from build123d import *

# Parameters (mm, degrees)
SKETCH_1_R          = 4
EXTRUDE_1_DEPTH     = 5
SKETCH_2_W          = 20.529114817
SKETCH_2_H          = 31.412366712
CUT_EXTRUDE_1_DEPTH = 5
EXTRUDE_2_DEPTH     = 20
SKETCH_4_W          = 7.585483435
SKETCH_4_H          = 20
EXTRUDE_3_DEPTH     = 10
SKETCH_5_W          = 7.585483435
SKETCH_5_H          = 20
SKETCH_5_W_2        = 3.706183356
EXTRUDE_4_DEPTH     = 5
SKETCH_6_W          = 3.75
SKETCH_6_H          = 12
CUT_EXTRUDE_2_DEPTH = 3
CUT_EXTRUDE_3_REACH = 54
SKETCH_7_R          = 1.275
FILLET_1_R          = 3
FILLET_2_R          = 1


with BuildPart() as part:
    # 草图1 → 凸台-拉伸1 (new body)
    with BuildSketch(Plane(origin=(0, 0, 0), x_dir=(1, 0, 0), z_dir=(0, 1, 0))):
        with BuildLine():
            Line((30, 40), (-30, 40))
            ThreePointArc((-30, 40), (-37.071067812, 37.071067812), (-40, 30))
            Line((-40, 30), (-40, -30))
            ThreePointArc((-40, -30), (-37.071067812, -37.071067812), (-30, -40))
            Line((-30, -40), (30, -40))
            ThreePointArc((30, -40), (37.071067812, -37.071067812), (40, -30))
            Line((40, -30), (40, 30))
            ThreePointArc((40, 30), (37.071067812, 37.071067812), (30, 40))
        make_face()
        with Locations((-30, 30)):
            Circle(SKETCH_1_R, mode=Mode.SUBTRACT)
        with Locations((-30, -30)):
            Circle(SKETCH_1_R, mode=Mode.SUBTRACT)
        with Locations((30, -30)):
            Circle(SKETCH_1_R, mode=Mode.SUBTRACT)
        with Locations((30, 30)):
            Circle(SKETCH_1_R, mode=Mode.SUBTRACT)
    extrude(amount=EXTRUDE_1_DEPTH)

    # 草图2 → 切除-拉伸1 (cut)
    with BuildSketch(Plane(origin=(0, 5, 0), x_dir=(1, 0, 0), z_dir=(0, 1, 0))):
        with Locations((-10.264557408, 0)):
            Rectangle(SKETCH_2_W, SKETCH_2_H)
    extrude(amount=-CUT_EXTRUDE_1_DEPTH, mode=Mode.SUBTRACT)

    # 草图3 → 凸台-拉伸2 (add)
    with BuildSketch(Plane(origin=(0, 5, 0), x_dir=(1, 0, 0), z_dir=(0, 1, 0))):
        with BuildLine():
            Line((0, -15.706183356), (-20.529114817, -15.706183356))
            Line((-20.529114817, -15.706183356), (-20.529114817, 15.706183356))
            Line((-20.529114817, 15.706183356), (0, 15.706183356))
            Line((0, 15.706183356), (0, 23.291666791))
            Line((0, 23.291666791), (-22.012764878, 23.291666791))
            ThreePointArc((-22.012764878, 23.291666791), (-25.548298784, 21.827200697), (-27.012764878, 18.291666791))
            Line((-27.012764878, 18.291666791), (-27.012764878, -18.291666791))
            ThreePointArc((-27.012764878, -18.291666791), (-25.548298784, -21.827200697), (-22.012764878, -23.291666791))
            Line((-22.012764878, -23.291666791), (0, -23.291666791))
            Line((0, -23.291666791), (0, -15.706183356))
        make_face()
    extrude(amount=EXTRUDE_2_DEPTH)

    # 草图4 → 凸台-拉伸3 (add)
    with BuildSketch(Plane(origin=(0, 0, 0), x_dir=(0, 0, -1), z_dir=(1, 0, 0))):
        with Locations((19.498925074, 15)):
            Rectangle(SKETCH_4_W, SKETCH_4_H)
        with Locations((-19.498925074, 15)):
            Rectangle(SKETCH_4_W, SKETCH_4_H)
    extrude(amount=EXTRUDE_3_DEPTH)

    # 草图5 → 凸台-拉伸4 (add, symmetric)
    with BuildSketch(Plane(origin=(10, 0, 0), x_dir=(0, 0, -1), z_dir=(1, 0, 0))):
        with Locations((-19.498925074, 15)):
            Rectangle(SKETCH_5_W, SKETCH_5_H)
        with Locations((-13.853091678, 15)):
            Rectangle(SKETCH_5_W_2, SKETCH_5_H)
        with Locations((13.853091678, 15)):
            Rectangle(SKETCH_5_W_2, SKETCH_5_H)
        with Locations((19.498925074, 15)):
            Rectangle(SKETCH_5_W, SKETCH_5_H)
    extrude(amount=EXTRUDE_4_DEPTH, both=True)

    # 草图6 → 切除-拉伸2 (cut)
    with BuildSketch(Plane(origin=(15, 0, 0), x_dir=(0, 0, -1), z_dir=(1, 0, 0))):
        with Locations((-13.875, 15)):
            Rectangle(SKETCH_6_W, SKETCH_6_H)
        with Locations((13.875, 15)):
            Rectangle(SKETCH_6_W, SKETCH_6_H)
    extrude(amount=-CUT_EXTRUDE_2_DEPTH, mode=Mode.SUBTRACT)

    # 草图7 → 切除-拉伸3 (cut, up to next)
    with BuildSketch(Plane(origin=(12, 0, 0), x_dir=(0, 0, -1), z_dir=(1, 0, 0)), mode=Mode.PRIVATE) as cut_extrude_3_sk1:
        with Locations((-13.91, 15)):
            Circle(SKETCH_7_R)
    cut_extrude_3_tool1 = extrude(cut_extrude_3_sk1.sketch, amount=-CUT_EXTRUDE_3_REACH, mode=Mode.PRIVATE) & part.part
    add(cut_extrude_3_tool1.solids().sort_by_distance((12, 15, 13.91))[0], mode=Mode.SUBTRACT)
    # 草图7 → 切除-拉伸3 (cut, up to next)
    with BuildSketch(Plane(origin=(12, 0, 0), x_dir=(0, 0, -1), z_dir=(1, 0, 0)), mode=Mode.PRIVATE) as cut_extrude_3_sk2:
        with Locations((13.91, 15)):
            Circle(SKETCH_7_R)
    cut_extrude_3_tool2 = extrude(cut_extrude_3_sk2.sketch, amount=-CUT_EXTRUDE_3_REACH, mode=Mode.PRIVATE) & part.part
    add(cut_extrude_3_tool2.solids().sort_by_distance((12, 15, -13.91))[0], mode=Mode.SUBTRACT)

    # 圆角1
    fillet_1_edges = [part.edges().sort_by_distance(p)[0] for p in [
        (15, 25, 17.645833395),
        (15, 15, 23.291666791),
        (15, 25, -17.645833395),
        (15, 15, -23.291666791),
        (-27.012764878, 25, 0),
        (-25.548298784, 25, 21.827200697),
        (-3.506382439, 25, 23.291666791),
        (-3.506382439, 25, -23.291666791),
        (-25.548298784, 25, -21.827200697),
    ]]
    fillet(fillet_1_edges, radius=FILLET_1_R)

    # 圆角2
    fillet_2_edges = [part.edges().sort_by_distance(p)[0] for p in [
        (37.071067812, 5, -37.071067812),
        (0, 5, -40),
        (-37.071067812, 5, -37.071067812),
        (-40, 5, 0),
        (-37.071067812, 5, 37.071067812),
        (0, 5, 40),
        (37.071067812, 5, 37.071067812),
        (40, 5, 0),
    ]]
    fillet(fillet_2_edges, radius=FILLET_2_R)


solid = part.part
Work out the finished part from the listing and answer in its coordinate system (mm). A direction names the side the tool comes from. Give positions to 0.01 mm unless a question says otherwise; leave off trailing zeros. Loops run counter-clockwise (first coordinate to the right, second up) from the corner with the lowest first, then second, coordinate; pieces in that order, holes last. Notation, with made-up numbers: (6, 71) -> (49, 71) arc R14 ccw to (49, 82) -> close; hole circle Ø10 at (0, 63). An arc over 180 degrees is marked (long way). Use a Markdown table: item, result. Add a question column.
1) The part is cut by section D-D, the plane z = -3. Determine the outline of the cut face in (x, y), plus the area to 3 significant figures.
2) For a pull along X with two mould halves and no side action, classify faces 6 (the flat face through (14, 21, 14)), 7 (the cylindrical face through (-26.111, 24.145, 0.256)), 8 (the flat face through (-20.529, 12, 0)), 9 (the flat face through (12, 16.4, 14.3)) as +X half, -X half, draft (parallel to the pull), parting line (faces both ways), or undercut.
3) Which of the six approach directions +Z, -Z, +X, -X, +Y, -Y give full straight-line access (tool end or side, diameter ignored) to faces 1 (the flat face through (5, 15.1, 15.5)), 2 (the flat face through (14, 21, -14)), 3 (the flat face through (0, 2, 40)), 4 (the cylindrical face through (14.145, 13.619, -22.39)), 5 (the cylindrical face through (14.1, 24.14, 16.2))?
4) The part is cut by section C-C, the plane z = -13.91. Determine the outline of the cut face in (x, y) (3 decimals).
5) Each of these flat-tipped pins is pushed along its axis until it touches: P1, Ø4, axis at y = 19, z = 0.5, coming from the +X side; P2, Ø8, axis at x = -3, y = 15.5, coming from the +Z side; P3, Ø1.5, axis at x = 14, z = -14, coming from the +Y side. Where does it stop, or does it pass through?
6) The part is cut by section B-B, the plane x = -2. Determine the outline of the cut face in (y, z).
7) The part is cut by section A-A, the plane y = 15. Determine the outline of the cut face in (x, z) (3 decimals).
8) Consider line 1 along Z through (x, y) = (30, 2.5); line 2 along Z through (x, y) = (1, 9). Determine where each line is inside the solid, lowest interval first.
Reported:
| question | item | result |
|---|---|---|
| 1 | outline | (-40, 0) -> (-20.53, 0) -> (-20.53, 25) -> (-24.01, 25) arc R3 ccw to (-27.01, 22) -> (-27.01, 5) -> (-39, 5) arc R1 ccw to (-40, 4) -> close; (0, 0) -> (40, 0) -> (40, 4) arc R1 ccw to (39, 5) -> (0, 5) -> close |
| 1 | area | 425 mm^2 |
| 2 | face 6 | draft |
| 2 | face 7 | -X half |
| 2 | face 8 | undercut |
| 2 | face 9 | +X half |
| 3 | face 1 | +Y |
| 3 | face 2 | +X |
| 3 | face 3 | +Z, +X, -X, +Y, -Y |
| 3 | face 4 | -Z, +X, +Y |
| 3 | face 5 | +Z, -Z, +X, +Y |
| 4 | outline | (-40, 0) -> (-20.529, 0) -> (-20.529, 25) -> (-24.013, 25) arc R3 ccw to (-27.013, 22) -> (-27.013, 5) -> (-39, 5) arc R1 ccw to (-40, 4) -> close; (0, 0) -> (40, 0) -> (40, 4) arc R1 ccw to (39, 5) -> (15, 5) -> (15, 9) -> (12, 9) -> (12, 13.725) -> (5, 13.725) -> (5, 5) -> (0, 5) -> close; (5, 16.275) -> (12, 16.275) -> (12, 21) -> (15, 21) -> (15, 22) arc R3 ccw to (12, 25) -> (5, 25) -> close |
| 5 | P1 | stops at x = -20.53 |
| 5 | P2 | stops at z = 23.29 |
| 5 | P3 | stops at y = 24.73 |
| 6 | outline | (0, -40) -> (4, -40) arc R1 ccw to (5, -39) -> (5, -23.29) -> (22, -23.29) arc R3 ccw to (25, -20.29) -> (25, -15.71) -> (0, -15.71) -> close; (0, 15.71) -> (25, 15.71) -> (25, 20.29) arc R3 ccw to (22, 23.29) -> (5, 23.29) -> (5, 39) arc R1 ccw to (4, 40) -> (0, 40) -> close |
| 7 | outline | (-27.013, -18.292) arc R5 ccw to (-22.013, -23.292) -> (12, -23.292) arc R3 ccw to (15, -20.292) -> (15, -15.75) -> (12, -15.75) -> (12, -15.185) -> (5, -15.185) -> (5, -15.706) -> (-20.529, -15.706) -> (-20.529, 15.706) -> (5, 15.706) -> (5, 15.185) -> (12, 15.185) -> (12, 15.75) -> (15, 15.75) -> (15, 20.292) arc R3 ccw to (12, 23.292) -> (-22.013, 23.292) arc R5 ccw to (-27.013, 18.292) -> close; (5, -12.635) -> (12, -12.635) -> (12, -12) -> (5, -12) -> close; (5, 12) -> (12, 12) -> (12, 12.635) -> (5, 12.635) -> close |
| 8 | line 1 | z = -40 to -34, -26 to 26, 34 to 40 |
| 8 | line 2 | z = -23.29 to -15.71, 15.71 to 23.29 |
